Geometry: see drawing. Coordinates: mm, zero at the bounding-box minimum. Coordinates: 2 decimals unless noted, no trailing zeros. Order: outer loops, then holes, each group sorted by start corner. A loop starts at its lowest first (then second) coordinate and runs counter-clockwise, first axis right, second up. Notation, with made-up numbers: M -27.75,84 L -0.75,84 A18 cw -0.75,93 Z; hole C 86.25,77 d7. An arc over 180 degrees is marked long. One line per item, written item: value.
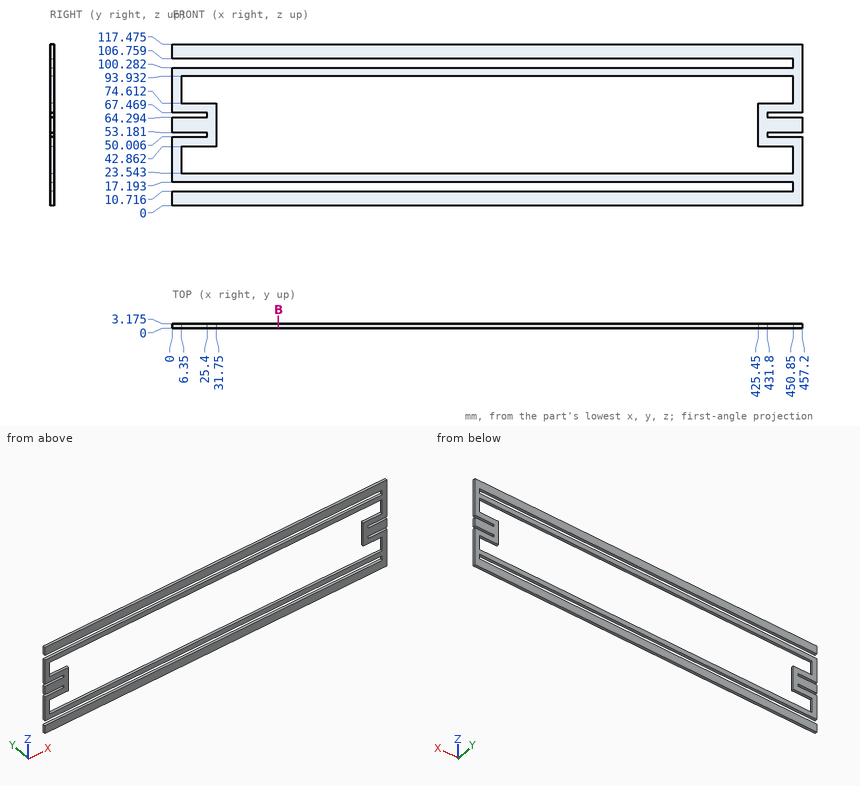
(1) Ray query, line 1 (Z direction, x = 233.5, y = 0.7) (1 decimal); line 2 (X direction, y = 1.5, z = 80.5); line 3 (X direction, y = 2, z = 43.5). Return the intervals inside material, ascending. Write a range as from..to.
Data:
line 1: z = 0..10.7, 17.2..23.5, 93.9..100.3, 106.8..117.5
line 2: x = 0..6.35, 450.85..457.2
line 3: x = 0..31.75, 425.45..457.2
(2) Cut plane B-B on x = 77. Output: boundary loops of the cut face in (y, z) (1 decimal).
Data:
outline: M 0,0 L 3.2,0 L 3.2,10.7 L 0,10.7 Z; M 0,17.2 L 3.2,17.2 L 3.2,23.5 L 0,23.5 Z; M 0,93.9 L 3.2,93.9 L 3.2,100.3 L 0,100.3 Z; M 0,106.8 L 3.2,106.8 L 3.2,117.5 L 0,117.5 Z
(3) First-contact query: pin 1 (1.6 mm diameter, centred on y = 1, z = 65.5, fed in from +X); pin 2 (1 mm diameter, centred on y = 1.5, z = 51, fed in from -X). Flat tips, straight axial feed; report the tip coordinate or a pass-through.
Data:
pin 1: stops at x = 431.8
pin 2: stops at x = 25.4
